Could you check a few things on this model? Use its own coordinates, in mm. A direction names the side the tool comes from. Give positions to 0.01 mm unless a question says otherwise; leave off trailing zeros. Order: outer loops, then holes, each group sorted by start corner. A loop starts at its lowest first (then second) coordinate and runs counter-clockwise, first axis right, second up.
from build123d import *

# Parameters (mm, degrees)
F0_R     = 2
F1_DEPTH = 5
F3_DEPTH = 2.5
F4_SIZE  = 1


with BuildPart() as f1:
    # F0 (on Top) → F1 (new body, symmetric)
    with BuildSketch(Plane.XY):
        Polygon((8.660254, 5), (0, 10), (-8.660254, 5), (-8.660254, -5), (0, -10), (8.660254, -5), align=None)
        Circle(F0_R, mode=Mode.SUBTRACT)
    extrude(amount=F1_DEPTH, both=True)

    # F2 (on Top) → F3 (join, symmetric)
    with BuildSketch(Plane.XY):
        Polygon((10.660254, -3), (10.660254, 0), (10.660254, 3), (8.660254, 3), (8.660254, 0), (8.660254, -3), align=None)
        Polygon((7.928203, 7.732051), (5.330127, 9.232051), (2.732051, 10.732051), (1.732051, 9), (4.330127, 7.5), (6.928203, 6), align=None)
        Polygon((-2.732051, 10.732051), (-5.330127, 9.232051), (-7.928203, 7.732051), (-6.928203, 6), (-4.330127, 7.5), (-1.732051, 9), align=None)
        Polygon((-10.660254, 3), (-10.660254, 0), (-10.660254, -3), (-8.660254, -3), (-8.660254, 0), (-8.660254, 3), align=None)
        Polygon((-7.928203, -7.732051), (-5.330127, -9.232051), (-2.732051, -10.732051), (-1.732051, -9), (-4.330127, -7.5), (-6.928203, -6), align=None)
        Polygon((2.732051, -10.732051), (5.330127, -9.232051), (7.928203, -7.732051), (6.928203, -6), (4.330127, -7.5), (1.732051, -9), align=None)
    extrude(amount=F3_DEPTH, both=True)

    # F4
    f4_edges = [f1.edges().sort_by_distance(p)[0] for p in [
        (10.660254, 3, 0),
        (10.660254, -3, 0),
        (7.928203, -7.732051, 0),
        (2.732051, -10.732051, 0),
        (-2.732051, -10.732051, 0),
        (-7.928203, -7.732051, 0),
        (-10.660254, -3, 0),
        (-10.660254, 3, 0),
        (-7.928203, 7.732051, 0),
        (-2.732051, 10.732051, 0),
        (2.732051, 10.732051, 0),
        (7.928203, 7.732051, 0),
    ]]
    chamfer(f4_edges, length=F4_SIZE)


solid = f1.part
Item 1: Imagine slicing it at C-C on x = -2.5. List the corners of the cut face in (y, z) for me.
Findings:
outline: (-9.94, -2.5) - (-8.56, -2.5) - (-8.56, -5) - (8.56, -5) - (8.56, -2.5) - (9.94, -2.5) - (9.94, 2.5) - (8.56, 2.5) - (8.56, 5) - (-8.56, 5) - (-8.56, 2.5) - (-9.94, 2.5) - close
Item 2: For faces 4 (the flat face through (8.66, 0, 3)), 5 (the flat face through (7.175, 6.427, -0.035)), 6 (the flat face through (1.98, -9.43, 0.04)), 7 (the flat face through (10, 0, 2.5)), 8 (the flat face through (5, -9, -2.5)), which set-ups out of +Z, -Z, +X, -X, +Y, -Y let a thin tool reach every point of the face, with its end or its side?
Findings:
face 4: +X
face 5: +Z, -Z, +X
face 6: +Z, -Z, -Y
face 7: +Z, +X, +Y, -Y
face 8: -Z, +X, -Y
Item 3: Imagine slicing it at A-A on y = -1. List the corners of the cut face in (x, z) for me.
Findings:
outline: (-10.66, -2.5) - (-8.66, -2.5) - (-8.66, -5) - (-1.73, -5) - (-1.73, 5) - (-8.66, 5) - (-8.66, 2.5) - (-10.66, 2.5) - close; (1.73, -5) - (8.66, -5) - (8.66, -2.5) - (10.66, -2.5) - (10.66, 2.5) - (8.66, 2.5) - (8.66, 5) - (1.73, 5) - close
Item 4: For pin 1 (1.1 mm diameter, centred on x = -9.5, z = -1, fed in from +Y); pin 2 (1.6 mm diameter, centred on x = -10, y = 1, fed in from -Z); pin 3 (1.6 mm diameter, centred on x = 9.5, y = 1, fed in from +Z); pin 4 (2 mm diameter, centred on x = -8.5, y = -6.5, fed in from -Z), each with a flat end and sliding along its axis, tell me the tip position at first contact or that it passes through.
Findings:
pin 1: stops at y = 3
pin 2: stops at z = -2.5
pin 3: stops at z = 2.5
pin 4: passes through
Item 5: We'd pull the mould along X, two halves only. Please class faces 1 (the flat face through (-10.66, 0, 0)), 2 (the flat face through (2.92, 10.05, -0.03)), 3 (the flat face through (-5, -9, 2.5)): +X half, -X half, draft (parallel to the pull), parting line (faces both ways), or undercut.
Findings:
face 1: -X half
face 2: undercut
face 3: draft
Item 6: Imagine slicing it at D-D on y = 7.5. List the corners of the cut face in (x, z) for me, then the cut area to 3 significant figures.
Findings:
outline: (-7.26, -2.5) - (-4.33, -2.5) - (-4.33, -5) - (4.33, -5) - (4.33, -2.5) - (7.26, -2.5) - (7.26, 2.5) - (4.33, 2.5) - (4.33, 5) - (-4.33, 5) - (-4.33, 2.5) - (-7.26, 2.5) - close
area: 116 mm2
Item 7: Imagine slicing it at B-B on x = 1.25. List the corners of the cut face in (y, z) for me.
Findings:
outline: (-9.28, -5) - (-1.56, -5) - (-1.56, 5) - (-9.28, 5) - close; (1.56, -5) - (9.28, -5) - (9.28, 5) - (1.56, 5) - close
Item 8: Please list where these lines run through material, in increasing order: line 1 along X through (y, z) = (2.25, 3.5); line 2 along Y through (x, z) = (7, 2.25); line 3 along Z through (x, y) = (-5.5, 8).
Findings:
line 1: x = -8.66 to 8.66
line 2: y = -8.27 to -6.12, -5.96 to 5.96, 6.12 to 8.27
line 3: z = -2.5 to 2.5
